Autodesk Inventor part; units mm, degrees
ref_plane "YZ Plane" through (0, 0, 0) normal (1, 0, 0) x (0, 1, 0)
ref_plane "XZ Plane" through (0, 0, 0) normal (0, 1, 0) x (-1, 0, 0)
ref_plane "XY Plane" through (0, 0, 0) normal (0, 0, 1) x (1, 0, 0)
sketch "Эскиз1" plane through (0, 0, 0) normal (0, 1, 0) x (-1, 0, 0)
  circle A0 centre (0, 0) radius 42
  line L0 (0, -42) -> (0, 42) construction
  circle A1 centre (18.0767, -25) radius 9
  circle A2 centre (-18.0767, -25) radius 9
  line L1 (39.598, -14) -> (-39.598, -14)
  circle A3 centre (0, -30.8507) radius 9
  circle A4 centre (0, 0) radius 30.8507 construction
  line L2 (0, 0) -> (12.9332, -39.9591) construction
  line L3 (0, 0) -> (-12.9332, -39.9591) construction
  line L4 (9.9159, -38.7553) -> (14.673, -37.2156)
  line L5 (14.673, -37.2156) -> (15.2888, -39.1184)
  line L6 (15.2888, -39.1184) -> (10.5318, -40.6581)
  line L7 (10.5318, -40.6581) -> (9.9159, -38.7553)
  line L8 (9.9159, -38.7553) -> (15.2888, -39.1184) construction
  line L9 (14.673, -37.2156) -> (10.5318, -40.6581) construction
  line L10 (-14.673, -37.2156) -> (-9.9159, -38.7553)
  line L11 (-9.9159, -38.7553) -> (-10.5318, -40.6581)
  line L12 (-10.5318, -40.6581) -> (-15.2888, -39.1184)
  line L13 (-15.2888, -39.1184) -> (-14.673, -37.2156)
  line L14 (-14.673, -37.2156) -> (-10.5318, -40.6581) construction
  line L15 (-9.9159, -38.7553) -> (-15.2888, -39.1184) construction
  line L16 (-2.5, -16.8507) -> (2.5, -16.8507)
  line L17 (2.5, -16.8507) -> (2.5, -18.8507)
  line L18 (2.5, -18.8507) -> (-2.5, -18.8507)
  line L19 (-2.5, -18.8507) -> (-2.5, -16.8507)
  line L20 (-2.5, -16.8507) -> (2.5, -18.8507) construction
  line L21 (2.5, -16.8507) -> (-2.5, -18.8507) construction
  circle A5 centre (0, 0) radius 17.0352
  circle A6 centre (0, 2) radius 44 construction
  circle A7 centre (31.1127, -29.1127) radius 2.5
  circle A8 centre (-31.1127, -29.1127) radius 2.5
  point P0 (12.6024, -38.9369)
  point P1 (-12.6024, -38.9369)
  point P2 (0, -17.8507)
  point P3 (9.7056, -14)
  point P4 (2.5, -16.8507)
  point P5 (-9.7056, -14)
  point P6 (-15.2888, -39.1184)
  point P7 (10.5318, -40.6581)
  point P8 (28.9734, -30.4063)
  point P9 (32.2615, -26.8923)
  point P10 (-32.2615, -26.8923)
  point P11 (-28.9734, -30.4063)
  dimension "d0" = 84
  dimension "d5" = 18
  dimension "d7" = 14
  dimension "d8" = 11
  dimension "d9" = 19
  dimension "d13" = 35.87
  dimension "d14" = 17.935
  dimension "d15" = 2
  dimension "d16" = 2
  dimension "d17" = 5
  dimension "d18" = 5
  dimension "d19" = 5
  dimension "d20" = 2
  dimension "d21" = 13
  dimension "d26" = 2
  dimension "d27" = 88
  dimension "d28" = 5
  dimension "d29" = 90
extrude "Выдавливание2" add sketch "Эскиз1" along normal blind 3 contours L1 A5 L19 L18 L17 A0 A7 L5 L4 L7 L11 L10 L13 A8
fillet "Сопряжение1" radius 10 2 edges at (-39.598, 1.5, -14) (39.598, 1.5, -14)
fillet "Сопряжение2" radius 10 2 edges at (-9.7056, 1.5, -14) (9.7056, 1.5, -14)
fillet "Сопряжение3" radius 5 4 edges at (28.9734, 1.5, -30.4063) (32.2615, 1.5, -26.8923) (-28.9734, 1.5, -30.4063) (-32.2615, 1.5, -26.8923)
equation "\"d14\" = 0.5 * d13"
properties part number "Крепление АКБ" material "Пластик АБС"
Design review of the part built by this model. Coordinates are the model's own, in mm. A direction names the side the tool comes from. Coordinates: 2 decimals unless noted, no trailing zeros. Order: outer loops, then holes, each group sorted by start corner. A loop starts at its lowest first (then second) coordinate and runs counter-clockwise, first axis right, second up. Notation, with made-up numbers: M -0.5,75.5 L 19.5,75.5 A9 cw 19.5,80.5 Z; hole C -13,78 d11. An arc over 180 degrees is marked long. Answer as a JSON object with one key per item and string values. Group by question number.
1) Mouldability with a two-part tool opening along Z and no side actions: class faces 4 (the flat face through (17, 1, -14)), 5 (the flat face through (10.22, 1.48, -39.69)), 6 (the cylindrical face through (-29.006, 1.479, -27.766)), 7 (the flat face through (0.5, 0, -21.6)) as pulls with the +Z half, pulls with the -Z half, needs draft (parallel to the pull), parting line crosses it, or undercut.
2) Tool access review of faces 1 (the cylindrical face through (9.49, 1.48, -27.7)), 2 (the flat face through (0, 1, -18.851)), 3 (the flat face through (14.985, 1.479, -38.18)): name each direction out of +Z, -Z, +X, -X, +Y, -Y from which nothing blocks a thin tool from reaching the whole face with its end or side.
3) Add section D-D, the plane y = 1.45. Count the separate pieces of the cut face and the enclosed holes in it, then the cut area to 3 significant figures.
4) Add section A-A, the plane x = 0. Write out the cut boundary in (y, z), then the cut area to 3 significant figures.
5) Wall thickness on L1, parallel to X at y = 2.4, z = -21.5; L2, parallel to X at y = 0.2, z = -33; L3, parallel to X at y = 2.7, z = -31.5: over which ranges is each line inside the solid? List them lowest first.
6) Add section C-C, the plane z = -18.25. Write out the cut boundary in (x, y).
7) For pin 1 (1.5 mm diameter, centred on x = -23.5, y = 0.5, fed in from -Z); pin 2 (11 mm diameter, centred on x = 0, z = -30.85, fed in from -Y); pin 3 (1.5 mm diameter, centred on x = 1, y = 2, fed in from -Z); pin 4 (1 mm diameter, centred on x = 2.5, y = 2, fed in from +Z), all flat-tipped, find the tip position at first contact; note any pin that passes through.
8) Add section B-B, the plane z = -35. Write out the cut boundary in (x, y).
Computed values:
{
 "1": {"face 4": "pulls with the +Z half", "face 5": "undercut", "face 6": "pulls with the -Z half", "face 7": "needs draft"},
 "2": {"face 1": "+Y, -Y", "face 2": "+Z, +Y, -Y", "face 3": "-Z, +Y, -Y"},
 "3": {"separate pieces": "1", "enclosed holes": "3", "area": "621 mm^2"},
 "4": {"outline": "M 0,-42 L 3,-42 L 3,-39.85 L 0,-39.85 Z; M 0,-21.85 L 3,-21.85 L 3,-18.85 L 0,-18.85 Z", "area": "15.4 mm^2"},
 "5": {"L1": "x = -32.36 to -26.37, -9.79 to 9.79, 26.37 to 32.36", "L2": "x = -25.98 to -22.2, -13.95 to -8.74, 8.74 to 13.95, 22.2 to 25.98", "L3": "x = -27.61 to -24.3, -11.85 to -8.98, 8.98 to 11.85, 24.3 to 27.61"},
 "6": {"outline": "M -30.87,0 L -24.03,0 L -24.03,3 L -30.87,3 Z; M -12.12,0 L -2.5,0 L -2.5,3 L -12.12,3 Z; M 2.5,0 L 12.12,0 L 12.12,3 L 2.5,3 Z; M 24.03,0 L 30.87,0 L 30.87,3 L 24.03,3 Z"},
 "7": {"pin 1": "stops at z = -35.3", "pin 2": "passes through", "pin 3": "stops at z = -42", "pin 4": "stops at z = -16.77"},
 "8": {"outline": "M -23.22,0 L -7.99,0 L -7.99,3 L -23.22,3 Z; M 7.99,0 L 23.22,0 L 23.22,3 L 7.99,3 Z"}
}
